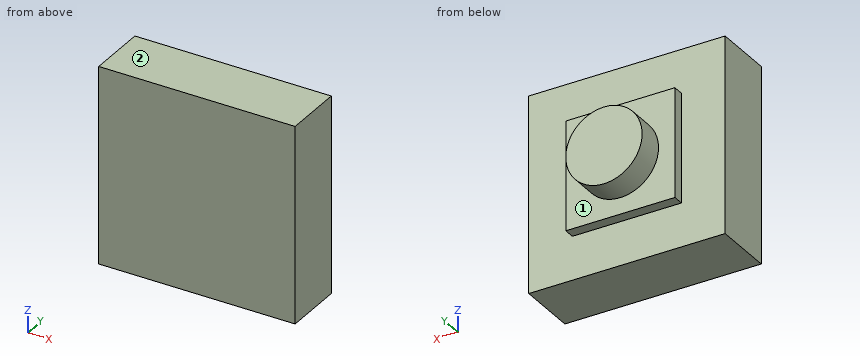
from build123d import *

# Parameters (mm, degrees)
SKETCH_1_W      = 36
SKETCH_1_H      = 36
EXTRUDE_1_DEPTH = 11
SKETCH_2_W      = 20
SKETCH_2_H      = 20
EXTRUDE_2_DEPTH = 2
SKETCH_4_R      = 7
EXTRUDE_4_DEPTH = 5


with BuildPart() as part:
    # 草图1 → 凸台-拉伸1 (new body)
    with BuildSketch(Plane(origin=(0, 0, 0), x_dir=(1, 0, 0), z_dir=(0, 1, 0))):
        Rectangle(SKETCH_1_W, SKETCH_1_H)
    extrude(amount=EXTRUDE_1_DEPTH)

    # 草图2 → 凸台-拉伸2 (add)
    with BuildSketch(Plane(origin=(0, 11, 0), x_dir=(1, 0, 0), z_dir=(0, 1, 0))):
        Rectangle(SKETCH_2_W, SKETCH_2_H)
    extrude(amount=EXTRUDE_2_DEPTH)

    # 草图4 → 凸台-拉伸4 (add)
    with BuildSketch(Plane(origin=(0, 13, 0), x_dir=(1, 0, 0), z_dir=(0, 1, 0))):
        with Locations(Location((0, 0, 0), (0, 0, 270))):
            Circle(SKETCH_4_R)
    extrude(amount=EXTRUDE_4_DEPTH)


solid = part.part
The model under review builds one solid part; all positions refer to its coordinate system, in mm. Face numbers are marked on the shaded views. A direction names the side the tool comes from. Give positions to 0.01 mm unless a question says otherwise; leave off trailing zeros. Order: outer loops, then holes, each group sorted by start corner. A loop starts at its lowest first (then second) coordinate and runs counter-clockwise, first axis right, second up. Notation, with made-up numbers: M 0,10.25 L 22,10.25 A23 ccw 22,36.25 Z; hole C -19.75,-4.5 d2. An arc over 180 degrees is marked long. One line per question, with ' | ' between items. Start each with the question number.
1) Consider section A-A, the plane x = 0. Give the boundary of the cut face in (y, z), then the cut area to 3 significant figures.
2) For the marked faces 1 and 2, list the 3-axis set-ups (+Z, -Z, +X, -X, +Y, -Y) from which the entire face can be reached by the end or side of a thin tool; tool diameter is ignored.
3) Clearance check with flat-ended pins moving along their axes: P1, Ø1, axis at x = -9, z = 2.5, coming from the +Y side; P2, Ø1.6, axis at y = 12, z = -0.5, coming from the +X side; P3, Ø5, axis at x = 11, y = 15, coming from the +Z side. State where each tip first meets the part, or that it passes through.
4) Consider section C-C, the plane x = 9. Give the boundary of the cut face in (y, z), then the cut area to 3 significant figures.
5) Consider section B-B, the plane z = 0. Give the boundary of the cut face in (x, y), then the cut area to 3 significant figures.
6) Wall thickness on L1, parallel to X at y = 11.75, z = -2; L2, parallel to Y at x = -4.5, z = -8.5; L3, parallel to Y at x = -11.5, z = -11: over which ranges is each line inside the solid? List them lowest first. Write a range as from..to.
7) Consider section D-D, the plane y = 16. Give the boundary of the cut face in (x, z), then the cut area to 3 significant figures.
Found:
1) outline: M 0,-18 L 11,-18 L 11,-10 L 13,-10 L 13,-7 L 18,-7 L 18,7 L 13,7 L 13,10 L 11,10 L 11,18 L 0,18 Z | area: 506 mm²
2) face 1: +Y | face 2: +Z, +X, -X, +Y, -Y
3) P1: stops at y = 13 | P2: stops at x = 10 | P3: stops at z = 10
4) outline: M 0,-18 L 11,-18 L 11,-10 L 13,-10 L 13,10 L 11,10 L 11,18 L 0,18 Z | area: 436 mm²
5) outline: M -18,0 L 18,0 L 18,11 L 10,11 L 10,13 L 7,13 L 7,18 L -7,18 L -7,13 L -10,13 L -10,11 L -18,11 Z | area: 506 mm²
6) L1: x = -10..10 | L2: y = 0..13 | L3: y = 0..11
7) outline: C 0,0 d14 | area: 154 mm²
